The model under review builds one solid part; all positions refer to its coordinate system, in mm. Face numbers are marked on the shaded views. Coordinates: 2 decimals unless noted, no trailing zeros. Order: outer loops, then holes, each group sorted by start corner. A loop starts at its lowest first (then second) coordinate and runs counter-clockwise, first axis right, second up. Notation, with made-up numbers: M -2,63 L 40,63 A8 ccw 40,67 Z; hole C 46,-24.75 d8. An arc over 180 degrees is marked long. One line per item, written item: value.
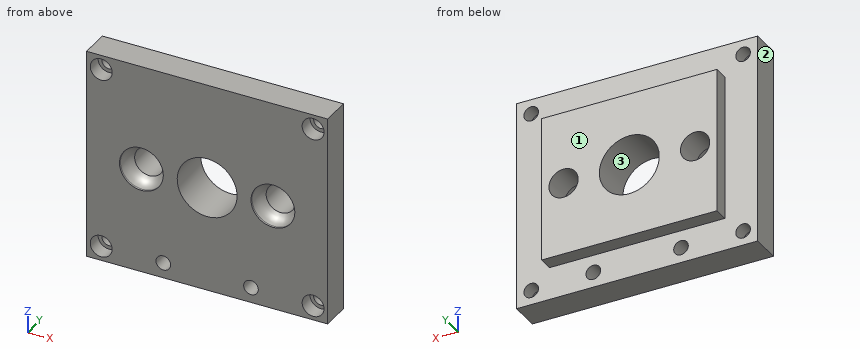
```python
from build123d import *

# Parameters (mm, degrees)
SKETCH_1_W          = 16.5
SKETCH_1_H          = 14.5
EXTRUDE_1_DEPTH     = 2
SKETCH_2_W          = 12
SKETCH_2_H          = 10
EXTRUDE_2_DEPTH     = 1
SKETCH_3_R          = 0.5
CUT_EXTRUDE_1_DEPTH = 12.163556781
SKETCH_5_R          = 2.05
SKETCH_5_R_2        = 1
CUT_EXTRUDE_2_DEPTH = 12.385297537
SKETCH_6_R          = 0.75
CUT_EXTRUDE_3_DEPTH = 1
SKETCH_7_R          = 1.5
CUT_EXTRUDE_4_DEPTH = 1
FILLET_1_R          = 1
SKETCH_8_R          = 0.5
CUT_EXTRUDE_5_DEPTH = 12.163556781


with BuildPart() as part:
    # 草图1 → 凸台-拉伸1 (new body)
    with BuildSketch(Plane(origin=(0, 0, 0), x_dir=(1, 0, 0), z_dir=(0, 1, 0))):
        Rectangle(SKETCH_1_W, SKETCH_1_H)
    extrude(amount=EXTRUDE_1_DEPTH)

    # 草图2 → 凸台-拉伸2 (add)
    with BuildSketch(Plane(origin=(0, 2, 0), x_dir=(1, 0, 0), z_dir=(0, 1, 0))):
        Rectangle(SKETCH_2_W, SKETCH_2_H)
    extrude(amount=EXTRUDE_2_DEPTH)

    # 草图3 → 切除-拉伸1 (cut, through all)
    with BuildSketch(Plane(origin=(0, 2, 0), x_dir=(1, 0, 0), z_dir=(0, 1, 0))):
        with Locations(Location((-7.25, 6.25, 0), (0, 0, 270))):
            Circle(SKETCH_3_R)
        with Locations(Location((7.25, 6.25, 0), (0, 0, 90))):
            Circle(SKETCH_3_R)
        with Locations(Location((7.25, -6.25, 0), (0, 0, 270))):
            Circle(SKETCH_3_R)
        with Locations(Location((-7.25, -6.25, 0), (0, 0, 90))):
            Circle(SKETCH_3_R)
    extrude(amount=-CUT_EXTRUDE_1_DEPTH, mode=Mode.SUBTRACT)

    # 草图5 → 切除-拉伸2 (cut, through all)
    with BuildSketch(Plane(origin=(0, 3, 0), x_dir=(1, 0, 0), z_dir=(0, 1, 0))):
        with Locations(Location((0, 0, 0), (0, 0, 270))):
            Circle(SKETCH_5_R)
        with Locations(Location((-4.5, 0, 0), (0, 0, 270))):
            Circle(SKETCH_5_R_2)
        with Locations(Location((4.5, 0, 0), (0, 0, 90))):
            Circle(SKETCH_5_R_2)
    extrude(amount=-CUT_EXTRUDE_2_DEPTH, mode=Mode.SUBTRACT)

    # 草图6 → 切除-拉伸3 (cut)
    with BuildSketch(Plane.XZ):
        with Locations(Location((7.25, -6.25, 0), (0, 0, 270))):
            Circle(SKETCH_6_R)
        with Locations(Location((-7.25, -6.25, 0), (0, 0, 270))):
            Circle(SKETCH_6_R)
        with Locations(Location((7.25, 6.25, 0), (0, 0, 270))):
            Circle(SKETCH_6_R)
        with Locations(Location((-7.25, 6.25, 0), (0, 0, 270))):
            Circle(SKETCH_6_R)
    extrude(amount=-CUT_EXTRUDE_3_DEPTH, mode=Mode.SUBTRACT)

    # 草图7 → 切除-拉伸4 (cut)
    with BuildSketch(Plane.XZ):
        with Locations(Location((-4.5, 0, 0), (0, 0, 270))):
            Circle(SKETCH_7_R)
        with Locations(Location((4.5, 0, 0), (0, 0, 270))):
            Circle(SKETCH_7_R)
    extrude(amount=-CUT_EXTRUDE_4_DEPTH, mode=Mode.SUBTRACT)

    # 圆角1
    # the kernel refuses this fillet: 1 mm, written as the material it adds along each edge
    with BuildSketch(Plane(origin=(-4.5, 1, 0), x_dir=(0, 0, -1), z_dir=(-1, 0, 0))) as fillet_1_piece_1_section:
        with BuildLine():
            CenterArc((0.5, 0.866025404), FILLET_1_R, 300, 60)
            Line((1, 0), (1.01, -0.017320508))
            ThreePointArc((1.01, -0.017320508), (1.25, -0.02), (1.5, -0.02))
            Line((1.5, -0.02), (1.52, 0))
            Line((1.52, 0), (1.52, 0.866025404))
            Line((1.52, 0.866025404), (1.5, 0.866025404))
        make_face()
    fillet_1_piece_1 = revolve(axis=Axis((-4.5, 1, 0), (0, -1, 0)), mode=Mode.PRIVATE)
    fillet_1_piece_1 = fillet_1_piece_1 - Plane(origin=(-4.5, 0.639457319, 0), x_dir=(0, 0, 1), z_dir=(0, 1, 0)) * Cylinder(1, 7, mode=Mode.PRIVATE)
    add(fillet_1_piece_1)
    with BuildSketch(Plane(origin=(4.5, 1, 0), x_dir=(0, 0, -1), z_dir=(-1, 0, 0))) as fillet_1_piece_2:
        with BuildLine():
            CenterArc((0.5, 0.866025404), FILLET_1_R, 300, 60)
            Line((1, 0), (1.01, -0.017320508))
            ThreePointArc((1.01, -0.017320508), (1.25, -0.02), (1.5, -0.02))
            Line((1.5, -0.02), (1.52, 0))
            Line((1.52, 0), (1.52, 0.866025404))
            Line((1.52, 0.866025404), (1.5, 0.866025404))
        make_face()
    revolve(axis=Axis((4.5, 1, 0), (0, -1, 0)))

    # 草图8 → 切除-拉伸5 (cut, through all)
    with BuildSketch(Plane(origin=(0, 2, 0), x_dir=(1, 0, 0), z_dir=(0, 1, 0))):
        with Locations(Location((-3, 6.2, 0), (0, 0, 270))):
            Circle(SKETCH_8_R)
        with Locations(Location((3, 6.2, 0), (0, 0, 90))):
            Circle(SKETCH_8_R)
    extrude(amount=-CUT_EXTRUDE_5_DEPTH, mode=Mode.SUBTRACT)


solid = part.part
```
(1) We need section D-D, the plane z = -4. State the section outline as (x, y) points, plus the area to 3 significant figures.
Geometry results:
outline: M -8.25,0 L 8.25,0 L 8.25,2 L 6,2 L 6,3 L -6,3 L -6,2 L -8.25,2 Z
area: 45.0 mm2
(2) We need section B-B, the plane x = 0. State the section outline as (y, z) points.
Geometry results:
outline: M 0,-7.25 L 2,-7.25 L 2,-5 L 3,-5 L 3,-2.05 L 0,-2.05 Z; M 0,2.05 L 3,2.05 L 3,5 L 2,5 L 2,7.25 L 0,7.25 Z
(3) Mouldability with a two-part tool opening along X and no side actions: class the marked faces 1, 2 and 3 as +X half, -X half, draft (parallel to the pull), parting line (faces both ways), or undercut.
Geometry results:
face 1: draft
face 2: -X half
face 3: undercut
(4) We need section A-A, the plane z = 6.25. State the section outline as (x, y) points.
Geometry results:
outline: M -8.25,0 L -8,0 L -8,1 L -7.75,1 L -7.75,2 L -8.25,2 Z; M -6.75,1 L -6.5,1 L -6.5,0 L 6.5,0 L 6.5,1 L 6.75,1 L 6.75,2 L -6.75,2 Z; M 7.75,1 L 8,1 L 8,0 L 8.25,0 L 8.25,2 L 7.75,2 Z
(5) Insertion check: pin 1 Ø0.8 at (y, z) = (2.5, 0) entering from +X; pin 2 Ø2 at (x, z) = (7.25, -6.25) entering from +Y; pin 3 Ø1.2 at (x, z) = (-7.25, 6.25) entering from -Y. Each pin has a flat end and moves straight along its axis. Give the tip position at first contact, or say it passes through.
Geometry results:
pin 1: stops at x = 6
pin 2: stops at y = 2
pin 3: stops at y = 1
(6) We need section C-C, the plane y = 1.7. Count the separate pieces of the cut face and the enclosed holes in it, plus the area to 3 significant figures.
Geometry results:
separate pieces: 1
enclosed holes: 9
area: 215 mm2
(7) For L1, parallel to X at y = 0.5, z = 6.25; L2, parallel to X at y = 2.15, z = 0; L3, parallel to X at y = 0.45, z = -6.25, list the stretches that pass through material, from the lowest coordinate up.
Geometry results:
L1: x = -8.25 to -8, -6.5 to 6.5, 8 to 8.25
L2: x = -6 to -5.5, -3.5 to -2.05, 2.05 to 3.5, 5.5 to 6
L3: x = -8.25 to -8, -6.5 to -3.5, -2.5 to 2.5, 3.5 to 6.5, 8 to 8.25
